Source: three-view drawing plus pictorial views. Frame: mm from the lowest corner of the part. A direction names the side the tool comes from. Give positions to 0.01 mm unless a question says otherwise; leave off trailing zeros. Loops run counter-clockwise (first coordinate to the right, second up) from the corner with the lowest first, then second, coordinate; pieces in that order, holes last.
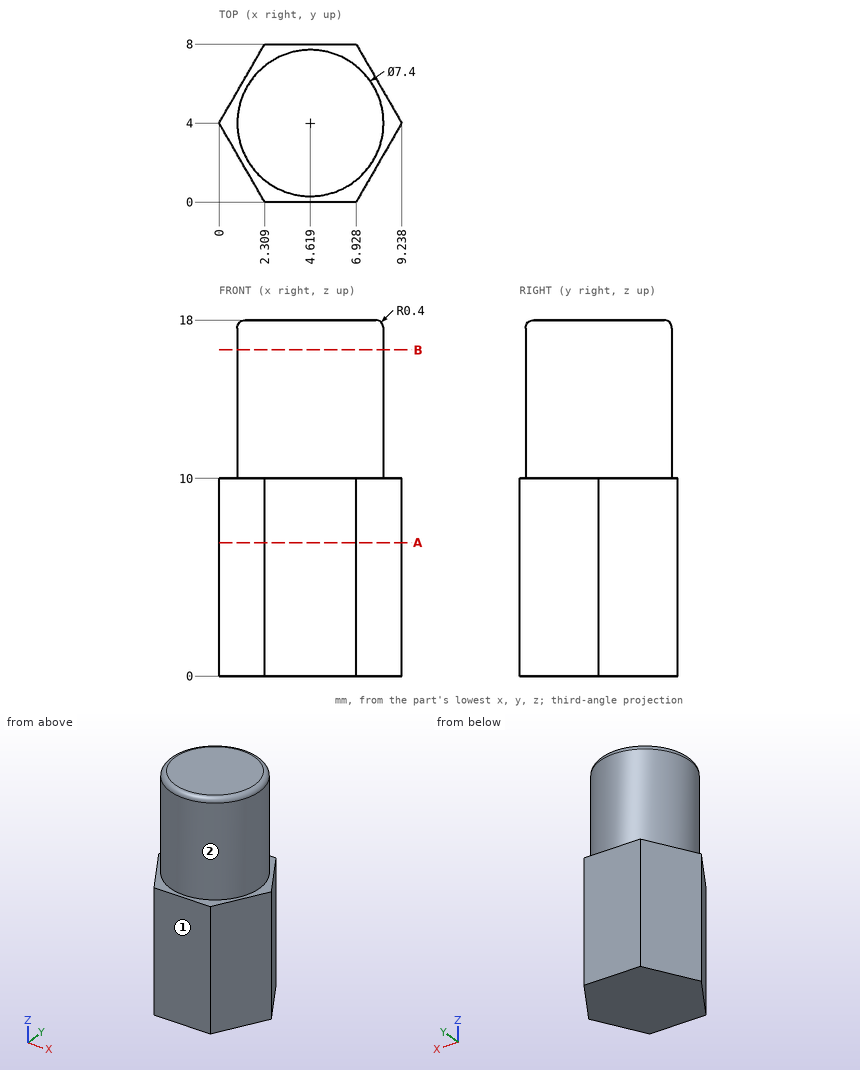
(1) Cut plane B-B (z = 16.5). Return the cut outline in (x, y), and give its area (3 significant figures).
Values follow:
outline: circle Ø7.4 at (4.62, 4)
area: 43.0 mm2
(2) Ray query, probe 1 along Z at (x, y) = (3, 0.5); probe 2 along Y at (x, z) = (7.25, 13.25); probe 3 along X at (y, z) = (5.75, 8). Return the intervals inside material, ascending.
Values follow:
probe 1: z = 0 to 10
probe 2: y = 1.4 to 6.6
probe 3: x = 1.01 to 8.23
(3) Reachability of the marked faces 1 and 2 from +Z, -Z, +X, -X, +Y, -Y: full face, straight path, thin tool, end or side. Return the list, or none.
Values follow:
face 1: +Z, -Z, +X, -X, -Y
face 2: +Z
(4) Cut plane A-A (z = 6.75). Return the cut outline in (x, y), and give its area (3 significant figures).
Values follow:
outline: (0, 4) - (2.31, 0) - (6.93, 0) - (9.24, 4) - (6.93, 8) - (2.31, 8) - close
area: 55.4 mm2
